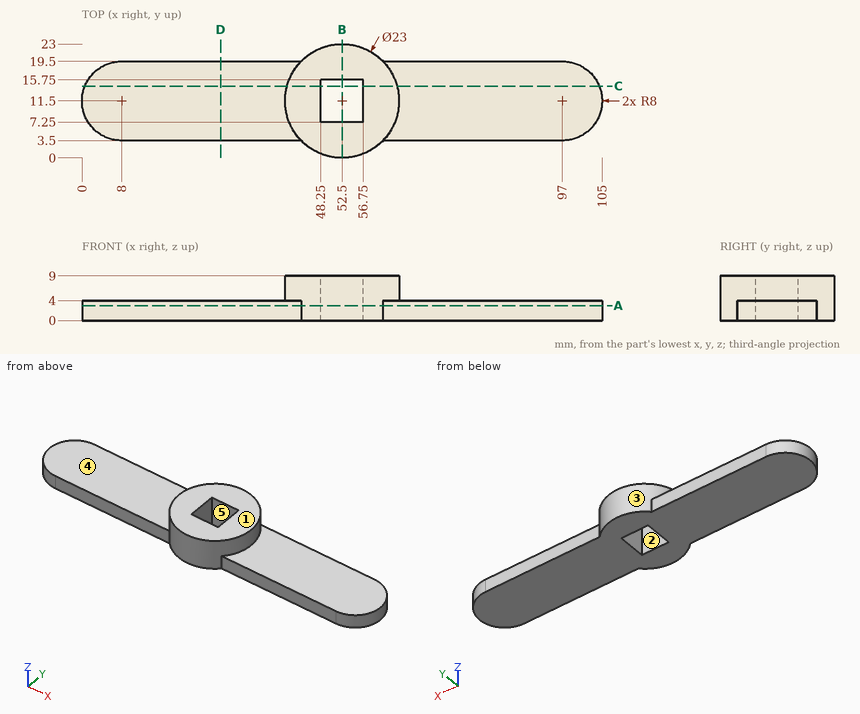
Answer from the drawing. Dimensions are ordinates in mm from the lowest x, y and z of the part. A direction names the side the tool comes from. Give positions to 0.01 mm unless a question says otherwise; leave off trailing zeros. Order: outer loops, then holes, each group sorted by start corner. A loop starts at its lowest first (then second) coordinate and runs counter-clockwise, first axis right, second up. Notation, with made-up numbers: (-9, 70.25) - (45, 70.25) arc R16 ccw to (45, 77.25) - close; hole circle Ø10 at (81.25, -12.5). An arc over 180 degrees is marked (long way). One line per item, written item: value. Start each with the question number.
1) Given pin 1 Ø4.5 at (x, z) = (18, 2) entering from +Y; pin 2 Ø2.5 at (x, z) = (51, 5.5) entering from +Y; pin 3 Ø4 at (x, y) = (26, 8) entering from +Z, each flat-ended and moving along its own axis, determine where each tip first touches the part or whether it passes through.
2) A cutting plane is placed at B-B on x = 52.5. Give the vertices of the cut face in (y, z).
3) The mould has two halves that part along X. Classify the marked faces 3, 4 and 5: released by +X, released by -X, zero draft, split by the parting line, or undercut.
4) A cutting plane is placed at D-D on x = 28. Give the vertices of the cut face in (y, z), then the cut area to 3 significant figures.
5) Find the intervals of material crossed by L1, parallel to Y at x = 53, z = 6.5; L2, parallel to Y at x = 68, z = 2; L3, parallel to Z at x = 89, y = 15.25, in increasing order.
6) A cutting plane is placed at C-C on y = 14.5. Give the vertices of the cut face in (x, z), then the cut area to 3 significant figures.
7) A tool of negligible diameter and unlimited length cuts with its end or side. For the marked faces 1 and 2, from which of +Z, -Z, +X, -X, +Y, -Y can it reach the whole face along a straight path? Write none if from no direction.
8) A cutting plane is placed at A-A on z = 3. Give the vertices of the cut face in (x, y), then the cut area to 3 significant figures.
Answer sheet:
1. pin 1: stops at y = 19.5
1. pin 2: stops at y = 23
1. pin 3: stops at z = 4
2. outline: (0, 0) - (7.25, 0) - (7.25, 9) - (0, 9) - close; (15.75, 0) - (23, 0) - (23, 9) - (15.75, 9) - close
3. face 3: split by the parting line
3. face 4: zero draft
3. face 5: undercut
4. outline: (3.5, 0) - (19.5, 0) - (19.5, 4) - (3.5, 4) - close
4. area: 64.0 mm2
5. L1: y = 0.01 to 7.25, 15.75 to 22.99
5. L2: y = 3.5 to 19.5
5. L3: z = 0 to 4
6. outline: (0.58, 0) - (48.25, 0) - (48.25, 9) - (41.4, 9) - (41.4, 4) - (0.58, 4) - close; (56.75, 0) - (104.42, 0) - (104.42, 4) - (63.6, 4) - (63.6, 9) - (56.75, 9) - close
6. area: 450 mm2
7. face 1: +Z, +X, -X, +Y, -Y
7. face 2: +Z, -Z
8. outline: (8, 3.5) - (44.24, 3.5) arc R11.5 ccw to (60.76, 3.5) - (97, 3.5) arc R8 ccw to (97, 19.5) - (60.76, 19.5) arc R11.5 ccw to (44.24, 19.5) - (8, 19.5) arc R8 ccw to start; hole (48.25, 7.25) - (56.75, 7.25) - (56.75, 15.75) - (48.25, 15.75) - close
8. area: 1,630 mm2
